from build123d import *

# Parameters (mm, degrees)
BOSS_EXTRUDE1_DEPTH = 1.905
SKETCH2_W           = 2.413
SKETCH2_H           = 6.858
CUT_EXTRUDE1_DEPTH  = 454.76030973


with BuildPart() as part:
    # Sketch1 → Boss-Extrude1 (new body)
    with BuildSketch(Plane.XY):
        with BuildLine():
            Line((-434.4289, 0), (-432.5239, 0))
            Line((-432.5239, 0), (-432.5239, -6.35))
            Line((-432.5239, -6.35), (-432.5239, -12.7))
            Line((-432.5239, -12.7), (-432.5239, -16.4084))
            ThreePointArc((-432.5239, -16.4084), (-433.669581115, -19.174318885), (-436.4355, -20.32))
            Line((-436.4355, -20.32), (-449.3895, -20.32))
            ThreePointArc((-449.3895, -20.32), (-452.155418885, -19.174318885), (-453.3011, -16.4084))
            Line((-453.3011, -16.4084), (-453.3011, -12.7))
            Line((-453.3011, -12.7), (-453.3011, -6.35))
            Line((-453.3011, -6.35), (-453.3011, 0))
            Line((-453.3011, 0), (-451.3961, 0))
            Line((-451.3961, 0), (-434.4289, 0))
        make_face()
    extrude(amount=BOSS_EXTRUDE1_DEPTH)

    # Sketch2 → Cut-Extrude1 (cut, through all)
    with BuildSketch(Plane.XY.offset(1.905)):
        with Locations((-433.4764, -9.525)):
            Rectangle(SKETCH2_W, SKETCH2_H)
        with Locations((-452.3486, -9.525)):
            Rectangle(SKETCH2_W, SKETCH2_H)
    extrude(amount=-CUT_EXTRUDE1_DEPTH, mode=Mode.SUBTRACT)


solid = part.part
Build history of the part. All positions in model axes, mm. A direction names the side the tool comes from. Round coordinates to 2 decimals unless told otherwise and drop trailing zeros. Loops run counter-clockwise (first coordinate to the right, second up) from the corner with the lowest first, then second, coordinate; pieces in that order, holes last. Notation, with made-up numbers: (41, 61) -> (86, 61) arc R15 ccw to (86, 69) -> close; hole circle Ø10 at (36, 29). An arc over 180 degrees is marked (long way). Use CSV: the item, a comma, the result in double quotes. Start each with the question number.
Q1. Saw through at C-C on y = -8. Give the cut face in (x, z) (3 decimals).
Q2. Flat gauge pins, fed straight in: pin 1 Ø1 at (x, z) = (-433.5, 1) entering from -Y; pin 2 Ø0.6 at (y, z) = (-10, 1) entering from +X; pin 3 Ø0.6 at (y, z) = (-11, 0.5) entering from -X. Where does each tip first touch, or does it go through?
Q3. Saw through at B-B on x = -433.75. Give the cut face in (y, z) (3 decimals).
Q4. Saw through at A-A on z = 1.5. Give the cut face in (x, y), and give its area (3 significant figures).
Q5. Mould opens along Y. For faces 4 (the face through (-443, -10, 1.905)), 5 (the face through (-443, -20.32, 1)), 6 (the face through (-434.683, -10, 1)), 7 (the face through (-451.142, -10, 1)) say: +Y half, -Y half, draft (parallel to the pull), parting line (faces both ways), or undercut.
Q6. Saw through at D-D on y = -19. Give the cut face in (x, z) (3 decimals).
Q7. Drill centre lines: L1, parallel to Y at x = -434.5, z = 0.6; L2, parallel to X at y = -6.25, z = 1.4; L3, parallel to X at y = -16.5, z = 1.5. Where is each one in solid material? Low to high.
Q8. Which spindle directions (+Z, -Z, +X, -X, +Y, -Y) get a long thin tool onto all of the face, cutting with end or side? Do faces 1 (the face through (-434, -12.954, 1)), 2 (the face through (-453.301, -3, 1)), 3 (the face through (-452, -12.954, 1)). Say none if no direction does.
Solutions:
1,outline,"(-451.142, 0) -> (-434.683, 0) -> (-434.683, 1.905) -> (-451.142, 1.905) -> close"
2,pin 1,"stops at y = -19.47"
2,pin 2,"stops at x = -434.68"
2,pin 3,"stops at x = -451.14"
3,outline,"(-19.252, 0) -> (-12.954, 0) -> (-12.954, 1.905) -> (-19.252, 1.905) -> close; (-6.096, 0) -> (0, 0) -> (0, 1.905) -> (-6.096, 1.905) -> close"
4,outline,"(-453.3, -16.41) arc R3.91 ccw to (-449.39, -20.32) -> (-436.44, -20.32) arc R3.91 ccw to (-432.52, -16.41) -> (-432.52, -12.95) -> (-434.68, -12.95) -> (-434.68, -6.1) -> (-432.52, -6.1) -> (-432.52, 0) -> (-453.3, 0) -> (-453.3, -6.1) -> (-451.14, -6.1) -> (-451.14, -12.95) -> (-453.3, -12.95) -> close"
4,area,"386 mm^2"
5,face 4,"draft"
5,face 5,"-Y half"
5,face 6,"undercut"
5,face 7,"undercut"
6,outline,"(-452.319, 0) -> (-433.506, 0) -> (-433.506, 1.905) -> (-452.319, 1.905) -> close"
7,L1,"y = -19.81 to -12.95, -6.1 to 0"
7,L2,"x = -451.14 to -434.68"
7,L3,"x = -453.3 to -432.52"
8,face 1,"+Z, -Z, +X"
8,face 2,"+Z, -Z, -X, +Y, -Y"
8,face 3,"+Z, -Z, -X"
